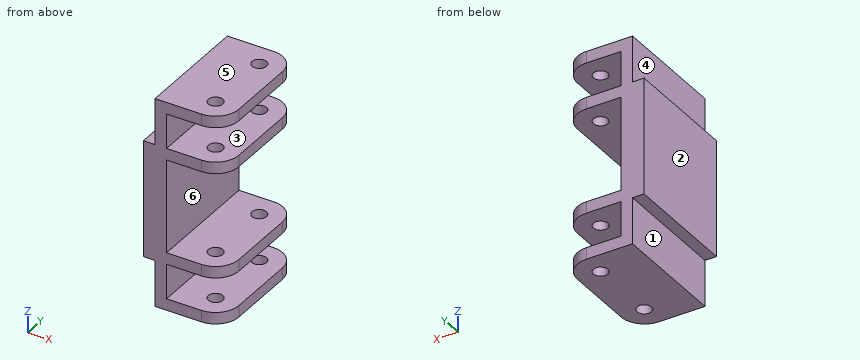
Autodesk Inventor part; units mm, degrees
ref_plane "YZ Plane" through (0, 0, 0) normal (1, 0, 0) x (0, 1, 0)
ref_plane "XZ Plane" through (0, 0, 0) normal (0, 1, 0) x (-1, 0, 0)
ref_plane "XY Plane" through (0, 0, 0) normal (0, 0, 1) x (1, 0, 0)
sketch "Sketch1" plane through (0, 0, 0) normal (1, 0, 0) x (0, 1, 0)
  line L0 (0, 0) -> (32, 0)
  line L1 (32, 0) -> (32, 32)
  line L2 (32, 32) -> (0, 32)
  line L3 (0, 32) -> (0, 0)
  dimension "d0" = 32
  dimension "d1" = 32
extrude "Extrusion1" add sketch "Sketch1" along normal blind 3.175
sketch "Sketch2" plane through (3.175, 0, 0) normal (1, 0, 0) x (0, 0, -1)
  line L0 (0, 32) -> (-32, 32)
  line L1 (-32, 0) -> (0, 0)
  line L2 (-32, 32) -> (-44.7, 32)
  line L3 (-44.7, 32) -> (-44.7, 0)
  line L4 (-44.7, 0) -> (-32, 0)
  line L5 (0, 32) -> (12.7, 32)
  line L6 (12.7, 32) -> (12.7, 0)
  line L7 (12.7, 0) -> (0, 0)
  dimension "d4" = 12.7
  dimension "d5" = 90
  dimension "d6" = 12.7
extrude "Extrusion2" add sketch "Sketch2" along normal blind 3.175
sketch "Sketch3" plane through (6.35, 0, 0) normal (1, 0, 0) x (0, 0, -1)
  line L0 (-32, 32) -> (-32, 0)
  line L1 (0, 0) -> (0, 32)
  line L2 (12.7, 0) -> (12.7, 32)
  line L3 (-44.7, 32) -> (-44.7, 0)
  line L4 (-32, 32) -> (-44.7, 32)
  line L5 (-44.7, 0) -> (-32, 0)
  line L6 (-44.7, 32) -> (-41.525, 32)
  line L7 (-41.525, 32) -> (-41.525, 0)
  line L8 (-41.525, 0) -> (-44.7, 0)
  line L9 (-44.7, 0) -> (-44.7, 32)
  line L10 (-32, 0) -> (0, 0)
  line L11 (-32, 32) -> (-28.825, 32)
  line L12 (-28.825, 32) -> (-28.825, 0)
  line L13 (-28.825, 0) -> (-32, 0)
  line L14 (-32, 0) -> (-32, 32)
  line L15 (0, 32) -> (-32, 32)
  line L16 (0, 32) -> (-3.175, 32)
  line L17 (-3.175, 32) -> (-3.175, 0)
  line L18 (-3.175, 0) -> (0, 0)
  line L19 (0, 0) -> (0, 32)
  line L20 (0, 0) -> (12.7, 0)
  line L21 (12.7, 32) -> (9.525, 32)
  line L22 (9.525, 32) -> (9.525, 0)
  line L23 (9.525, 0) -> (12.7, 0)
  line L24 (12.7, 0) -> (12.7, 32)
  dimension "d9" = 3.175
  dimension "d10" = 3.175
  dimension "d11" = 3.175
  dimension "d12" = 3.175
extrude "Extrusion3" add sketch "Sketch3" along normal blind 15.875 contours L11 L12 L10 L0 | L22 L21 L2 L20 | L7 L5 L3 L4 | L15 L1 L10 L17
fillet "Fillet1" radius 6.35 8 edges at (22.225, 32, 43.1125) (22.225, 32, 30.4125) (22.225, 0, 43.1125) (22.225, 0, 30.4125) (22.225, 0, 1.5875) (22.225, 32, 1.5875) (22.225, 32, -11.1125) (22.225, 0, -11.1125)
sketch "Sketch4" plane through (3.175, 0, 44.7) normal (0, 0, 1) x (1, 0, 0)
  arc A0 (19.05, 25.65) -> (12.7, 32) centre (12.7, 25.65) ccw
  arc A1 (12.7, 0) -> (19.05, 6.35) centre (12.7, 6.35) ccw
  point P0 (-3.175, 0)
hole "Hole1" at (15.875, 25.65, 44.7) at (15.875, 6.35, 44.7) direction (0, 0, -1) diameter 4 end through all
properties part number "pully mount"
Could you check a few things on this model? Use its own coordinates, in mm. Face numbers are marked on the shaded views. A direction names the side the tool comes from. Give positions to 0.01 mm unless a question says otherwise; leave off trailing zeros. Loops run counter-clockwise (first coordinate to the right, second up) from the corner with the lowest first, then second, coordinate; pieces in that order, holes last. Notation, with made-up numbers: (49, -14) - (92, -14) arc R35 cw to (92, 22) - close; hole circle Ø8 at (48, -13.75). An arc over 180 degrees is marked (long way). Use one line per item in the form item = value.
1. On a 3-axis mill with a long thin cutter (end or side, diameter ignored), from which of +Z, -Z, +X, -X, +Y, -Y can I reach the whole of each face in a straight line? I mean the marked faces 1, 2 and 3. Say none if no direction works.
Response values:
face_1 = -Z, -X, +Y, -Y
face_2 = +Z, -Z, -X, +Y, -Y
face_3 = +X, +Y, -Y
2. I want a section at D-D (x = 2). Please give me the cut outline in (y, z), and give its area (3 significant figures).
Response values:
outline = (0, 0) - (32, 0) - (32, 32) - (0, 32) - close
area = 1,020 mm²
3. I want a section at A-A (x = 11.5). Please give me the cut outline in (y, z) (3 decimals), and give its area (3 significant figures).
Response values:
outline = (0, -12.7) - (32, -12.7) - (32, -9.525) - (0, -9.525) - close; (0, 0) - (32, 0) - (32, 3.175) - (0, 3.175) - close; (0, 28.825) - (32, 28.825) - (32, 32) - (0, 32) - close; (0, 41.525) - (32, 41.525) - (32, 44.7) - (0, 44.7) - close
area = 406 mm²
4. I want a section at C-C (z = -6). Please give me the cut outline in (x, y) (3 decimals).
Response values:
outline = (3.175, 0) - (6.35, 0) - (6.35, 32) - (3.175, 32) - close
5. I want a section at B-B (y = 15). Please give me the cut outline in (x, z) (3 decimals), and give its area (3 significant figures).
Response values:
outline = (0, 0) - (3.175, 0) - (3.175, -12.7) - (22.225, -12.7) - (22.225, -9.525) - (6.35, -9.525) - (6.35, 0) - (22.225, 0) - (22.225, 3.175) - (6.35, 3.175) - (6.35, 28.825) - (22.225, 28.825) - (22.225, 32) - (6.35, 32) - (6.35, 41.525) - (22.225, 41.525) - (22.225, 44.7) - (3.175, 44.7) - (3.175, 32) - (0, 32) - close
area = 485 mm²
6. I need wall thicknesses on probe 1 along Z at (x, y) = (11.5, 23.5) (3 decimals); probe 2 along X at (y, z) = (6.35, -12) (3 decimals); probe 3 along Y at (x, z) = (16.5, 31). Which ranges of each line are inside material? Lowest first, please.
Response values:
probe_1 = -12.7 to -9.525, 0 to 3.175, 28.825 to 32, 41.525 to 44.7
probe_2 = 3.175 to 13.875, 17.875 to 22.225
probe_3 = 0.03 to 4.45, 8.25 to 23.75, 27.55 to 31.97
7. I'm going to push flat-ended pins straight in: pin 1 Ø1 at (x, y) = (2, 21.5) entering from +Z; pin 2 Ø10 at (y, z) = (15, -9) entering from -X (3 decimals); pin 3 Ø7.5 at (y, z) = (20, 16) entering from +X. Where does each tip first touch, or does it pass through?
Response values:
pin_1 = 32
pin_2 = 3.175
pin_3 = 6.35
8. Thinking about a two-plate mould opening in Z: for the marked faces 4, 5 and 6, which applies, released by +Z, released by -Z, zero draft, split by the parting line, or undercut?
Response values:
face_4 = zero draft
face_5 = released by +Z
face_6 = undercut
